The drawing under review shows one solid part. Ordinate dimensions are in mm from its lowest x, y, z. A direction names the side the tool comes from. Coordinates: 2 decimals unless noted, no trailing zeros. Loops run counter-clockwise (first coordinate to the right, second up) from the corner with the lowest first, then second, coordinate; pieces in that order, holes last. Notation, with made-up numbers: (4.25, 29) -> (26.25, 29) arc R15 ccw to (26.25, 35) -> close; hole circle Ø2 at (38, -13). An arc over 180 degrees is marked (long way). Use a Markdown table: item, result.
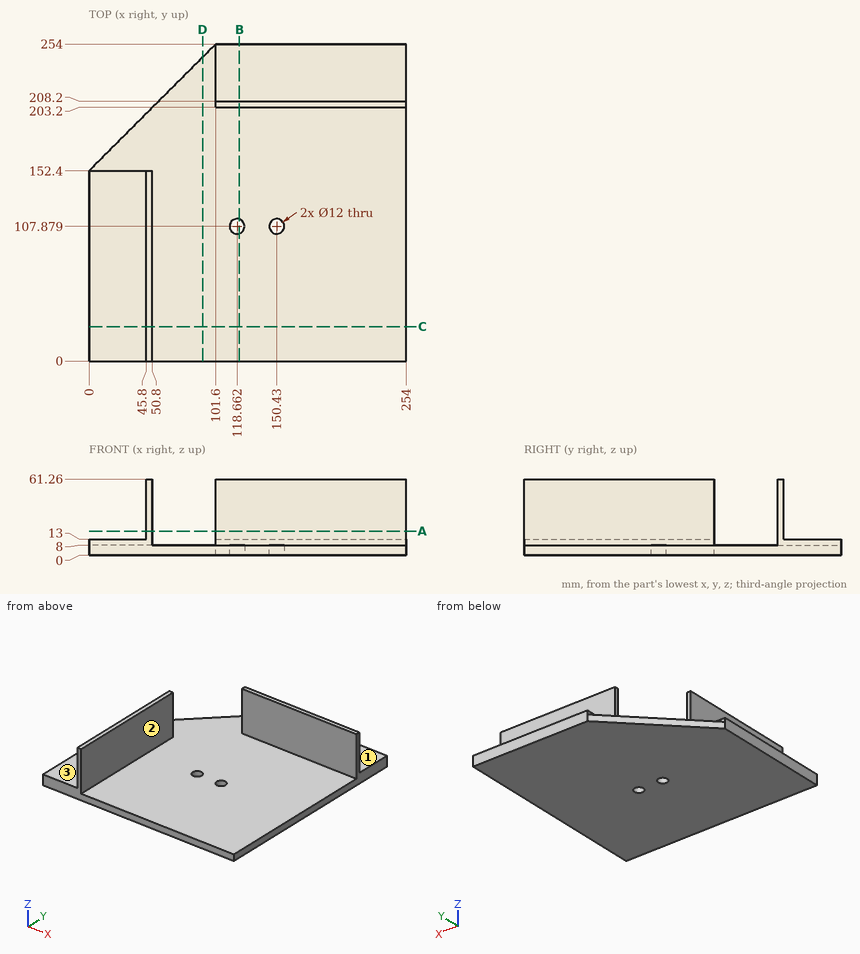
(1) For pin 1 Ø8 at (x, z) = (53, 30) entering from +Y; pin 2 Ø5 at (x, z) = (182, 20.5) entering from -Y; pin 3 Ø14.5 at (y, z) = (100.5, 38.5) entering from -X, all flat-tipped, find the tip position at first contact; note any pin that passes through.
Found:
| item | result |
|---|---|
| pin 1 | stops at y = 152.4 |
| pin 2 | stops at y = 203.2 |
| pin 3 | stops at x = 45.8 |
(2) Take a section at D-D on x = 91. Write out the cut boundary in (y, z).
Found:
| item | result |
|---|---|
| outline | (0, 0) -> (243.4, 0) -> (243.4, 8) -> (0, 8) -> close |
(3) For line 1 along X through (y, z) = (130, 47.5); line 2 along Z through (x, y) = (216, 215); line 3 along Z through (x, y) = (65, 154), list the stretches that pass through material, from the lowest coordinate up.
Found:
| item | result |
|---|---|
| line 1 | x = 45.8 to 50.8 |
| line 2 | z = 0 to 13 |
| line 3 | z = 0 to 8 |
(4) Take a section at A-A on z = 19.5. Write out the cut boundary in (x, y), plus the area to 3 significant figures.
Found:
| item | result |
|---|---|
| outline | (45.8, 0) -> (50.8, 0) -> (50.8, 152.4) -> (45.8, 152.4) -> close; (101.6, 203.2) -> (254, 203.2) -> (254, 208.2) -> (101.6, 208.2) -> close |
| area | 1,520 mm^2 |
(5) Take a section at C-C on y = 27.5. Write out the cut boundary in (x, z).
Found:
| item | result |
|---|---|
| outline | (0, 0) -> (254, 0) -> (254, 8) -> (50.8, 8) -> (50.8, 61.26) -> (45.8, 61.26) -> (45.8, 13) -> (0, 13) -> close |
(6) Take a section at B-B on x = 120.5. Write out the cut boundary in (y, z), plus the area to 3 significant figures.
Found:
| item | result |
|---|---|
| outline | (0, 0) -> (102.17, 0) -> (102.17, 8) -> (0, 8) -> close; (113.59, 0) -> (254, 0) -> (254, 13) -> (208.2, 13) -> (208.2, 61.26) -> (203.2, 61.26) -> (203.2, 8) -> (113.59, 8) -> close |
| area | 2,440 mm^2 |
(7) For the marked faces 1, 2 and 3, list the 3-axis set-ups (+Z, -Z, +X, -X, +Y, -Y) from which the entire face can be reached by the end or side of a thin tool; tool diameter is ignored.
Found:
| item | result |
|---|---|
| face 1 | +Z, +X, -X, +Y |
| face 2 | +Z, +X, +Y, -Y |
| face 3 | +Z, -X, +Y, -Y |
